from build123d import *

# Parameters (mm, degrees)
BOSS_EXTRUDE1_DEPTH        = 45
FILLET1_R                  = 30
CUT_EXTRUDE1_REACH         = 202.352
SKETCH2_R                  = 22
FILLET2_R                  = 30
M30X2_0_TAPPED_HOLE1_D     = 28
M30X2_0_TAPPED_HOLE1_DEPTH = 35
M30X2_0_TAPPED_HOLE1_TIP   = 8.412048666
SKETCH5_R                  = 7
CUT_EXTRUDE2_DEPTH         = 201.352189906
SKETCH6_W                  = 30
SKETCH6_H                  = 25
CUT_EXTRUDE3_DEPTH         = 10
FILLET3_R                  = 5
M6_TAPPED_HOLE1_AT_2_COUNT = 2
M6_TAPPED_HOLE1_AT_2_PITCH = 12
CUT_EXTRUDE4_REACH         = 202.352
SKETCH9_R                  = 4


# Read off the part's stored shape, not the designer's step: M8 Tapped Hole1, Ø8.0mm Dowel Hole1, M8 Tapped Hole2, Ø8.0mm Dowel Hole2
with BuildPart() as part:
    # Sketch1 → Boss-Extrude1 (new body)
    with BuildSketch(Plane(origin=(0, 0, 0), x_dir=(1, 0, 0), z_dir=(0, 1, 0))):
        with BuildLine():
            Line((-142.577164466, 53.422835534), (-115, 25.845671067))
            Line((-115, 25.845671067), (-115, -120))
            Line((-115, -120), (115, -120))
            Line((115, -120), (115, 25.845671067))
            Line((115, 25.845671067), (142.577164466, 53.422835534))
            ThreePointArc((142.577164466, 53.422835534), (142.577164466, 108.577164466), (87.422835534, 108.577164466))
            Line((87.422835534, 108.577164466), (59.845671067, 81))
            Line((59.845671067, 81), (-59.845671067, 81))
            Line((-59.845671067, 81), (-87.422835534, 108.577164466))
            ThreePointArc((-87.422835534, 108.577164466), (-142.577164466, 108.577164466), (-142.577164466, 53.422835534))
        make_face()
    extrude(amount=-BOSS_EXTRUDE1_DEPTH)

    # Fillet1
    fillet1_edges = [part.edges().sort_by_distance(p)[0] for p in [
        (-59.845671067, -22.5, -81),
        (59.845671067, -22.5, -81),
        (115, -22.5, -25.845671067),
        (-115, -22.5, -25.845671067),
    ]]
    fillet(fillet1_edges, radius=FILLET1_R)

    # Sketch2 → Cut-Extrude1 (cut, up to next)
    with BuildSketch(Plane(origin=(0, 0, 0), x_dir=(1, 0, 0), z_dir=(0, 1, 0)), mode=Mode.PRIVATE) as cut_extrude1_sk1:
        with Locations(Location((-115, 81, 0), (0, 0, 270))):
            Circle(SKETCH2_R)
    cut_extrude1_tool1 = extrude(cut_extrude1_sk1.sketch, amount=-CUT_EXTRUDE1_REACH, mode=Mode.PRIVATE) & part.part
    # Sketch2 → Cut-Extrude1 (cut, up to next)
    with BuildSketch(Plane(origin=(0, 0, 0), x_dir=(1, 0, 0), z_dir=(0, 1, 0)), mode=Mode.PRIVATE) as cut_extrude1_sk2:
        with Locations(Location((115, 81, 0), (0, 0, 270))):
            Circle(SKETCH2_R)
    cut_extrude1_tool2 = extrude(cut_extrude1_sk2.sketch, amount=-CUT_EXTRUDE1_REACH, mode=Mode.PRIVATE) & part.part
    add(cut_extrude1_tool1.solids().sort_by_distance((-115, 0, -81))[0], mode=Mode.SUBTRACT)
    add(cut_extrude1_tool2.solids().sort_by_distance((115, 0, -81))[0], mode=Mode.SUBTRACT)

    # Fillet2
    fillet2_edges = [part.edges().sort_by_distance(p)[0] for p in [
        (115, -22.5, 120),
        (-115, -22.5, 120),
    ]]
    fillet(fillet2_edges, radius=FILLET2_R)

    # M30x2.0 Tapped Hole1
    with Locations(Plane(origin=(0, 0, 0), x_dir=(1, 0, 0), z_dir=(0, 1, 0))):
        with Locations((0, -32.5)):
            Hole(M30X2_0_TAPPED_HOLE1_D / 2, depth=M30X2_0_TAPPED_HOLE1_DEPTH)
            with Locations((0, 0, -(M30X2_0_TAPPED_HOLE1_DEPTH + M30X2_0_TAPPED_HOLE1_TIP / 2))):  # 118° drill point
                Cone(0, M30X2_0_TAPPED_HOLE1_D / 2, M30X2_0_TAPPED_HOLE1_TIP, mode=Mode.SUBTRACT)

    # Sketch5 → Cut-Extrude2 (cut, through all)
    with BuildSketch(Plane(origin=(0, 0, 0), x_dir=(1, 0, 0), z_dir=(0, 1, 0))):
        with Locations(Location((-33.8, -32.5, 0), (0, 0, 270))):
            Circle(SKETCH5_R)
        with Locations(Location((4.2, -32.5, 0), (0, 0, 270))):
            Circle(SKETCH5_R)
    extrude(amount=-CUT_EXTRUDE2_DEPTH, mode=Mode.SUBTRACT)

    # Sketch6 → Cut-Extrude3 (cut)
    with BuildSketch(Plane.XZ.offset(45)):
        with Locations((-110, 32.5)):
            Rectangle(SKETCH6_W, SKETCH6_H)
    extrude(amount=-CUT_EXTRUDE3_DEPTH, mode=Mode.SUBTRACT)

    # Fillet3
    fillet3_edges = [part.edges().sort_by_distance(p)[0] for p in [
        (-95, -40, 45),
        (-95, -40, 20),
    ]]
    fillet(fillet3_edges, radius=FILLET3_R)

    # Sketch8 → M6 Tapped Hole1 (revolve, cut)
    with BuildSketch(Plane(origin=(-105, -35, 26.5), x_dir=(0, 0, -1), z_dir=(1, 0, 0))):
        Polygon((0, 0), (0, 35), (3.025, 35), (2.5, 34.475), (2.5, 0.525), (3.025, 0), align=None)
    m6_tapped_hole1 = revolve(axis=Axis((-105, -41.35, 26.5), (0, 1, 0)), mode=Mode.SUBTRACT)

    # M6 Tapped Hole1 at 2: M6 Tapped Hole1 ×2
    with Locations(*[(0, 0, i * M6_TAPPED_HOLE1_AT_2_PITCH) for i in range(1, M6_TAPPED_HOLE1_AT_2_COUNT)]):
        add(m6_tapped_hole1, mode=Mode.SUBTRACT)

    # Sketch9 → Cut-Extrude4 (cut, up to next)
    with BuildSketch(Plane(origin=(0, 0, 0), x_dir=(1, 0, 0), z_dir=(0, 1, 0)), mode=Mode.PRIVATE) as cut_extrude4_sk1:
        with Locations((-115.715161352, -32.5)):
            Circle(SKETCH9_R)
    cut_extrude4_tool1 = extrude(cut_extrude4_sk1.sketch, amount=-CUT_EXTRUDE4_REACH, mode=Mode.PRIVATE) & part.part
    add(cut_extrude4_tool1.solids().sort_by_distance((-115.715161, 0, 32.5))[0], mode=Mode.SUBTRACT)

    # M8 Tapped Hole1 outline → M8 Tapped Hole1 (revolve, cut)
    with BuildSketch(Plane(origin=(-56.8, 0, 59.5), x_dir=(1, 0, 0), z_dir=(0, 0, 1))):
        Polygon((4.025, 0), (0, 0), (0, -45), (4.025, -45), (3.4, -44.375), (3.4, -0.625), align=None)
    revolve(axis=Axis((-56.8, 0, 59.5), (0, 1, 0)), mode=Mode.SUBTRACT)

    # M8 Tapped Hole1 2 outline → M8 Tapped Hole1 2 (revolve, cut)
    with BuildSketch(Plane(origin=(3.2, 0, 59.5), x_dir=(1, 0, 0), z_dir=(0, 0, 1))):
        Polygon((4.025, 0), (0, 0), (0, -45), (4.025, -45), (3.4, -44.375), (3.4, -0.625), align=None)
    revolve(axis=Axis((3.2, 0, 59.5), (0, 1, 0)), mode=Mode.SUBTRACT)

    # M8 Tapped Hole1 3 outline → M8 Tapped Hole1 3 (revolve, cut)
    with BuildSketch(Plane(origin=(3.2, 0, 5.5), x_dir=(1, 0, 0), z_dir=(0, 0, 1))):
        Polygon((4.025, 0), (0, 0), (0, -45), (4.025, -45), (3.4, -44.375), (3.4, -0.625), align=None)
    revolve(axis=Axis((3.2, 0, 5.5), (0, 1, 0)), mode=Mode.SUBTRACT)

    # M8 Tapped Hole1 4 outline → M8 Tapped Hole1 4 (revolve, cut)
    with BuildSketch(Plane(origin=(-56.8, 0, 5.5), x_dir=(1, 0, 0), z_dir=(0, 0, 1))):
        Polygon((4.025, 0), (0, 0), (0, -45), (4.025, -45), (3.4, -44.375), (3.4, -0.625), align=None)
    revolve(axis=Axis((-56.8, 0, 5.5), (0, 1, 0)), mode=Mode.SUBTRACT)

    # Ø8.0mm Dowel Hole1 outline → Ø8.0mm Dowel Hole1 (revolve, cut)
    with BuildSketch(Plane(origin=(-39.8, 0, 59.5), x_dir=(1, 0, 0), z_dir=(0, 0, 1))):
        Polygon((0, -45), (4.025, -45), (4, -44.975), (4, -0.025), (4.025, 0), (0, 0), align=None)
    revolve(axis=Axis((-39.8, 0, 59.5), (0, 1, 0)), mode=Mode.SUBTRACT)

    # 8.0mm Dowel Hole1 2 outline → 8.0mm Dowel Hole1 2 (revolve, cut)
    with BuildSketch(Plane(origin=(-13.8, 0, 5.5), x_dir=(1, 0, 0), z_dir=(0, 0, 1))):
        Polygon((0, -45), (4.025, -45), (4, -44.975), (4, -0.025), (4.025, 0), (0, 0), align=None)
    revolve(axis=Axis((-13.8, 0, 5.5), (0, 1, 0)), mode=Mode.SUBTRACT)

    # M8 Tapped Hole2 outline → M8 Tapped Hole2 (revolve, cut)
    with BuildSketch(Plane(origin=(75.8, 0, 11.5), x_dir=(1, 0, 0), z_dir=(0, 0, 1))):
        Polygon((4.025, 0), (0, 0), (0, -45), (4.025, -45), (3.4, -44.375), (3.4, -0.625), align=None)
    revolve(axis=Axis((75.8, 0, 11.5), (0, 1, 0)), mode=Mode.SUBTRACT)

    # M8 Tapped Hole2 2 outline → M8 Tapped Hole2 2 (revolve, cut)
    with BuildSketch(Plane(origin=(33.8, 0, 53.5), x_dir=(1, 0, 0), z_dir=(0, 0, 1))):
        Polygon((4.025, 0), (0, 0), (0, -45), (4.025, -45), (3.4, -44.375), (3.4, -0.625), align=None)
    revolve(axis=Axis((33.8, 0, 53.5), (0, 1, 0)), mode=Mode.SUBTRACT)

    # Ø8.0mm Dowel Hole2 outline → Ø8.0mm Dowel Hole2 (revolve, cut)
    with BuildSketch(Plane(origin=(75.8, 0, 53.5), x_dir=(1, 0, 0), z_dir=(0, 0, 1))):
        Polygon((4.025, 0), (0, 0), (0, -45), (4.025, -45), (4, -44.975), (4, -0.025), align=None)
    revolve(axis=Axis((75.8, 0, 53.5), (0, 1, 0)), mode=Mode.SUBTRACT)

    # 8.0mm Dowel Hole2 2 outline → 8.0mm Dowel Hole2 2 (revolve, cut)
    with BuildSketch(Plane(origin=(33.8, 0, 11.5), x_dir=(1, 0, 0), z_dir=(0, 0, 1))):
        Polygon((4.025, 0), (0, 0), (0, -45), (4.025, -45), (4, -44.975), (4, -0.025), align=None)
    revolve(axis=Axis((33.8, 0, 11.5), (0, 1, 0)), mode=Mode.SUBTRACT)


solid = part.part
Design review of the part built by this model. Coordinates are the model's own, in mm. A direction names the side the tool comes from. Coordinates: 2 decimals unless noted, no trailing zeros. Loops run counter-clockwise (first coordinate to the right, second up) from the corner with the lowest first, then second, coordinate; pieces in that order, holes last. Notation, with made-up numbers: (3, 3.5) - (56, 3.5) arc R16 cw to (56, 9.5) - close; hole circle Ø6 at (9, -2). An arc over 180 degrees is marked (long way). Use CSV: the item, a comma, the result in double quotes. Start each with the question number.
1. Mouldability with a two-part tool opening along X and no side actions: class faces 3 (the flat face through (-95, -40, 32)), 4 (the flat face through (-105, -35, 33)), 5 (the cylindrical face through (-141.96, -22.18, -109.18)) as released by +X, released by -X, zero draft, split by the parting line, or undercut.
2. Add section C-C on z = -19. Give the boundary of the cut face in (x, y).
3. Clearance check with flat-ended pins moving along their axes: pin 1 (8 mm diameter, centred on y = -8, z = 66, fed in from -X); pin 2 (8 mm diameter, centred on x = 75.8, z = 11.5, fed in from -Y) (3 decimals); pin 3 (6 mm diameter, centred on y = -37.5, z = 73, fed in from +X). State where each tip first meets the part, or that it passes through.
4. Add section B-B on x = 119. Give the boundary of the cut face in (y, z).
5. Add section A-A on y = -23.5. Count the separate pieces of the cut face and the enclosed holes in it, plus the area to 3 significant figures.
6. For faces 1 (the flat face through (78.159, -22.185, -99.314)), 2 (the cylindrical face through (78.94, -22.19, 12.8)), list the 3-axis set-ups (+Z, -Z, +X, -X, +Y, -Y) from which the entire face can be reached by the end or side of a thin tool; tool diameter is ignored.
7. To check wall thickness, follow probe 1 along X at (y, z) = (-19, 5.5); probe 2 along X at (y, z) = (-24.5, 32.5); probe 3 along X at (y, z) = (-20, 53.5). State the ranges of each line that lie inside material, in increasing order.
Resolved:
1,face 3,"released by -X"
1,face 4,"zero draft"
1,face 5,"undercut"
2,outline,"(-115.52, -45) - (115.52, -45) - (115.52, 0) - (-115.52, 0) - close"
3,pin 1,"x = -115"
3,pin 2,"y = -44.975"
3,pin 3,"x = 115"
4,outline,"(-45, -119.79) - (0, -119.79) - (0, -102.63) - (-45, -102.63) - close; (-45, -59.37) - (0, -59.37) - (0, -28.39) - (-45, -28.39) - close"
5,separate pieces,"1"
5,enclosed holes,"16"
5,area,"49,500 mm2"
6,face 1,"-Z, +Y, -Y"
6,face 2,"+Y, -Y"
7,probe 1,"-115 to -60.2, -53.4 to -17.8, -9.8 to -0.2, 6.6 to 115"
7,probe 2,"-111.72 to -40.8, -26.8 to -14, 14 to 115"
7,probe 3,"-115 to 30.4, 37.2 to 71.8, 79.8 to 115"
